from build123d import *

# Parameters (mm, degrees)
F0_R     = 91.44
F0_R_2   = 78.74
F1_DEPTH = 5
F2_SIZE  = 1
F3_SIZE  = 1


with BuildPart() as f1:
    # F0 (on Front) → F1 (new body)
    with BuildSketch(Plane.XZ):
        with Locations((-18.093221, 4.894068)):
            Circle(F0_R)
        with Locations((-18.093221, 4.894068)):
            Circle(F0_R_2, mode=Mode.SUBTRACT)
    extrude(amount=F1_DEPTH)

    # F2
    f2_edges = [f1.edges().sort_by_distance(p)[0] for p in [
        (-109.533221, -5, 4.894068),
    ]]
    chamfer(f2_edges, length=F2_SIZE)

    # F3
    f3_edges = [f1.edges().sort_by_distance(p)[0] for p in [
        (-96.833221, -5, 4.894068),
    ]]
    chamfer(f3_edges, length=F3_SIZE)


solid = f1.part
Can you work these out from the model? Positions are in its coordinate system, mm. Give positions to 0.01 mm unless a question says otherwise; leave off trailing zeros. Order: outer loops, then holes, each group sorted by start corner. A loop starts at its lowest first (then second) coordinate and runs counter-clockwise, first axis right, second up. Notation, with made-up numbers: M -15.5,11 L 41.5,11 A23 cw 41.5,49 Z; hole C 50.25,61 d8. An arc over 180 degrees is marked long. Use one line per item in the form item = value. Start each with the question number.
Item 1: We'd pull the mould along X, two halves only. Please class faces 1 (the cylindrical face through (18.24, -1.97, -64.96)), 2 (the flat face through (22, 0, 73)), 3 (the cylindrical face through (-85.49, -1.97, 66.69)): +X half, -X half, draft (parallel to the pull), parting line (faces both ways), or undercut.
Item 2: Will this pin go through, and if not, where does the flat tip stop? pin 1 Ø1 at (x, y) = (12.5, -2.5) entering from -Z.
Item 3: If we section it at A-A (y = -2.3): Write out the boundary of the cut face in (x, z).
Item 4: If I drill on line 1 along X through (y, z) = (-2.65, 7.5); line 2 along Z through (x, y) = (37, -1.8); line 3 along X through (y, z) = (-2.2, -42.5), over which ranges is the centre line in solid material (lowest first)?
Outcome:
q1.face_1 = undercut
q1.face_2 = draft
q1.face_3 = parting line
q2.pin_1 = -81.45
q3.outline = C -18.09,4.89 d182.88; hole C -18.09,4.89 d157.48
q4.line_1 = -109.5 to -96.79, 60.6 to 73.31
q4.line_2 = -68.09 to -51.36, 61.15 to 77.87
q4.line_3 = -96.29 to -80.97, 44.79 to 60.11
